CAD build for the part. Positions are in the model's coordinates, mm. A direction names the side the tool comes from. Round coordinates to 2 decimals unless told otherwise and drop trailing zeros. Loops run counter-clockwise (first coordinate to the right, second up) from the corner with the lowest first, then second, coordinate; pieces in that order, holes last. Notation, with made-up numbers: M -31,59.5 L 9,59.5 A32 cw 9,93.5 Z; hole C 52.5,11.5 d9. An arc over 180 degrees is marked long. Use one line per item in the form item = value.
from build123d import *

# Parameters (mm, degrees)
SKETCH1_W           = 10
SKETCH1_H           = 10
SKETCH1_W_2         = 8
SKETCH1_H_2         = 8
BOSS_EXTRUDE1_DEPTH = 105
SKETCH2_R           = 2.125
CUT_EXTRUDE1_DEPTH  = 116
SKETCH4_R           = 2.125
CUT_EXTRUDE3_DEPTH  = 10


with BuildPart() as part:
    # Sketch1 → Boss-Extrude1 (new body)
    with BuildSketch(Plane.XY):
        with Locations((5, 5)):
            Rectangle(SKETCH1_W, SKETCH1_H)
        with Locations((5, 5)):
            Rectangle(SKETCH1_W_2, SKETCH1_H_2, mode=Mode.SUBTRACT)
    extrude(amount=BOSS_EXTRUDE1_DEPTH)

    # Sketch2 → Cut-Extrude1 (cut)
    with BuildSketch(Plane(origin=(0, 10, 0), x_dir=(1, 0, 0), z_dir=(0, 1, 0))):
        with Locations(Location((5, -5, 0), (0, 0, 270))):
            Circle(SKETCH2_R)
        with Locations(Location((5, -15, 0), (0, 0, 270))):
            Circle(SKETCH2_R)
        with Locations(Location((5, -100, 0), (0, 0, 270))):
            Circle(SKETCH2_R)
        with Locations(Location((5, -90, 0), (0, 0, 270))):
            Circle(SKETCH2_R)
    extrude(amount=-CUT_EXTRUDE1_DEPTH, mode=Mode.SUBTRACT)

    # Sketch4 → Cut-Extrude3 (cut)
    with BuildSketch(Plane(origin=(10, 0, 0), x_dir=(0, 0, -1), z_dir=(1, 0, 0))):
        with Locations((-70, 5)):
            Circle(SKETCH4_R)
        with Locations((-35, 5)):
            Circle(SKETCH4_R)
    extrude(amount=-CUT_EXTRUDE3_DEPTH, mode=Mode.SUBTRACT)


solid = part.part
1. Cut at A-A on y = 5. Write the cut outline in (x, z) (3 decimals).
Completed:
outline = M 0,0 L 1,0 L 1,32.875 L 0,32.875 Z; M 0,37.125 L 1,37.125 L 1,67.875 L 0,67.875 Z; M 0,72.125 L 1,72.125 L 1,105 L 0,105 Z; M 9,0 L 10,0 L 10,32.875 L 9,32.875 Z; M 9,37.125 L 10,37.125 L 10,67.875 L 9,67.875 Z; M 9,72.125 L 10,72.125 L 10,105 L 9,105 Z
2. Tool access for faces 4 (the face through (2.926, 0.507, 4.539)), 5 (the face through (5, 1, 52)): list every direction of +Z, -Z, +X, -X, +Y, -Y with a clear straight run to the whole face (end or side of a thin tool).
Completed:
face_4 = +Y, -Y
face_5 = +Z, -Z
3. Drop a flat-ended pin along its axis: P1, Ø2.5, axis at x = 5, z = 90, coming from the -Y side. Give the stop position or say it passes through.
Completed:
P1 = through
4. Cut at B-B on z = 35. Write the cut outline in (x, y) (3 decimals), and give its area (3 significant figures).
Completed:
outline = M 0,0 L 10,0 L 10,2.875 L 9,2.875 L 9,1 L 1,1 L 1,2.875 L 0,2.875 Z; M 0,7.125 L 1,7.125 L 1,9 L 9,9 L 9,7.125 L 10,7.125 L 10,10 L 0,10 Z
area = 27.5 mm2
5. Probe line 1 along X through (y, z) = (9.35, 90) (3 decimals); line 2 along X through (y, z) = (2, 42). List the from-to ranges inside material, lowest first. Write a range as from..to.
Completed:
line_1 = 0..2.875, 7.125..10
line_2 = 0..1, 9..10
6. Cut at C-C on z = 49.5. Write the cut outline in (x, y).
Completed:
outline = M 0,0 L 10,0 L 10,10 L 0,10 Z; hole M 1,1 L 9,1 L 9,9 L 1,9 Z
7. Pull direction Y, two halves, no side cores. Call faces 1 (the face through (1, 5, 52)), 2 (the face through (3.71, 9.51, 88.31)), 3 (the face through (5, 10, 52)): +Y half, -Y half, draft (parallel to the pull), parting line (faces both ways), or undercut.
Completed:
face_1 = undercut
face_2 = draft
face_3 = +Y half
